Can you work these out from the drawing? Everything is in mm from the part's minimum corner. A direction names the side the tool comes from. Round coordinates to 2 decimals unless told otherwise and drop trailing zeros. Loops run counter-clockwise (first coordinate to the right, second up) from the corner with the lowest first, then second, coordinate; pieces in that order, holes last. Notation, with made-up numbers: (-29.75, 73.25) -> (6.25, 73.25) arc R7 ccw to (6.25, 78.25) -> close; hole circle Ø10 at (-24.75, 84.5). An arc over 180 degrees is marked (long way). Answer as a JSON object with one key per item and string values.
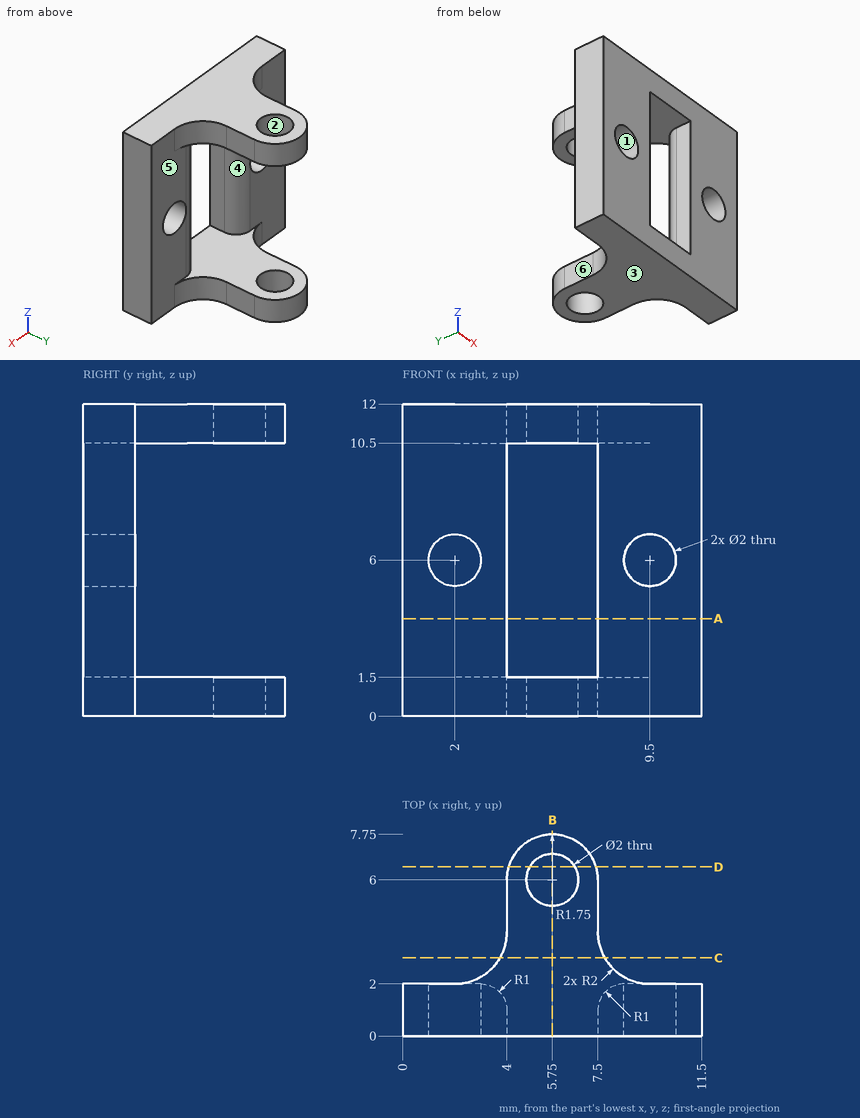
Q1. If I drill on L1, parallel to X at y = 0.95, z = 6; L2, parallel to Y at x = 5.75, z = 11.3; L3, parallel to Z at x = 6.5, y = 7, over which ranges is the centre line in solid material (lowest first)? Write a range as [from, to].
Determined:
{"L1": "[0, 1], [3, 4], [7.5, 8.5], [10.5, 11.5]", "L2": "[0, 5], [7, 7.75]", "L3": "[0, 1.5], [10.5, 12]"}
Q2. I want a section at D-D, the plane y = 6.5. Write out the boundary of the cut face in (x, z).
Determined:
{"outline": "(4.07, 0) -> (4.88, 0) -> (4.88, 1.5) -> (4.07, 1.5) -> close; (4.07, 10.5) -> (4.88, 10.5) -> (4.88, 12) -> (4.07, 12) -> close; (6.62, 0) -> (7.43, 0) -> (7.43, 1.5) -> (6.62, 1.5) -> close; (6.62, 10.5) -> (7.43, 10.5) -> (7.43, 12) -> (6.62, 12) -> close"}
Q3. I want a section at C-C, the plane y = 3. Write out the boundary of the cut face in (x, z).
Determined:
{"outline": "(3.73, 0) -> (7.77, 0) -> (7.77, 1.5) -> (3.73, 1.5) -> close; (3.73, 10.5) -> (7.77, 10.5) -> (7.77, 12) -> (3.73, 12) -> close"}
Q4. We'd pull the mould along Z, two halves only. Please class the marked faces 1, 2 and 3: pulls with the +Z half, pulls with the -Z half, needs draft (parallel to the pull), parting line crosses it, or undercut.
Determined:
{"face 1": "undercut", "face 2": "needs draft", "face 3": "pulls with the -Z half"}
Q5. On a 3-axis mill with a long thin cutter (end or side, diameter ignored), from which of +Z, -Z, +X, -X, +Y, -Y can I reach the whole of each face in a straight line? I mean the marked faces 4, 5 and 6. Say none if no direction works.
Determined:
{"face 4": "+Y", "face 5": "+X, +Y", "face 6": "+Z, -Z, -X, +Y"}
Q6. I'm going to push flat-ended pins straight in: pin 1 (0.8 mm diameter, centred on y = 5.5, z = 0.5, fed in from -X); pin 2 (2.5 mm diameter, centred on x = 2, z = 6, fed in from +Y); pin 3 (1.5 mm diameter, centred on x = 9, z = 1, fed in from +Y). Where does each tip first touch, or does it pass through?
Determined:
{"pin 1": "x = 4", "pin 2": "y = 2", "pin 3": "y = 2.44"}
Q7. I want a section at A-A, the plane z = 3.75. Write out the boundary of the cut face in (x, y).
Determined:
{"outline": "(0, 0) -> (4, 0) -> (4, 1) arc R1 ccw to (3, 2) -> (0, 2) -> close; (7.5, 0) -> (11.5, 0) -> (11.5, 2) -> (8.5, 2) arc R1 ccw to (7.5, 1) -> close"}
Q8. I want a section at B-B, the plane x = 5.75. Write out the boundary of the cut face in (y, z).
Determined:
{"outline": "(0, 0) -> (5, 0) -> (5, 1.5) -> (0, 1.5) -> close; (0, 10.5) -> (5, 10.5) -> (5, 12) -> (0, 12) -> close; (7, 0) -> (7.75, 0) -> (7.75, 1.5) -> (7, 1.5) -> close; (7, 10.5) -> (7.75, 10.5) -> (7.75, 12) -> (7, 12) -> close"}
